```python
from build123d import *

# Parameters (mm, degrees)
BOSS_EXTRUDE1_DEPTH = 10.16
SKETCH5_W           = 63.5
SKETCH5_H           = 20.32
CUT_EXTRUDE1_DEPTH  = 2126.25967614


with BuildPart() as part:
    # Sketch1 → Boss-Extrude1 (new body)
    with BuildSketch(Plane.XY):
        Polygon((-123.444, 2072.64), (-205.715298803, 2072.64), (-205.715298803, 2052.32), (-215.881789204, 2052.32), (-215.881789204, 1963.42), (-205.715298803, 1963.42), (-205.715298803, 1874.52), (-215.881789204, 1874.52), (-215.881789204, 1785.62), (-205.715298803, 1785.62), (-205.715298803, 1696.72), (-215.875298803, 1696.72), (-215.875298803, 1607.82), (-205.715298803, 1607.82), (-205.715298803, 1518.92), (-215.881789204, 1518.92), (-215.881789204, 1488.440000035), (-469.881789204, 1488.440000035), (-469.881789204, 0), (-375.428294602, 0), (-375.428294602, 20.32), (-280.9748, 20.32), (-280.9748, 0), (280.9748, 0), (280.9748, 20.32), (375.428294602, 20.32), (375.428294602, 0), (469.881789204, 0), (469.881789204, 1488.440000035), (215.881789204, 1488.440000035), (215.881789204, 1518.92), (205.715298803, 1518.92), (205.715298803, 1607.82), (215.875298803, 1607.82), (215.875298803, 1696.72), (205.715298803, 1696.72), (205.715298803, 1785.62), (215.881789204, 1785.62), (215.881789204, 1874.52), (205.715298803, 1874.52), (205.715298803, 1963.42), (215.881789204, 1963.42), (215.881789204, 2052.32), (205.715298803, 2052.32), (205.715298803, 2072.64), (123.444, 2072.64), (123.444, 2052.32), (41.135649402, 2052.32), (41.135649402, 2072.64), (-41.135649402, 2072.64), (-41.135649402, 2052.32), (-123.444, 2052.32), align=None)
        Polygon((215.881789204, 1463.040000035), (222.040744894, 1374.366931824), (211.92306481, 1373.664189215), (205.715298803, 1463.040000035), align=None, mode=Mode.SUBTRACT)
        Polygon((-205.715298803, 1463.040000035), (-211.92306481, 1373.664189215), (-222.040744894, 1374.366931824), (-215.881789204, 1463.040000035), align=None, mode=Mode.SUBTRACT)
        Polygon((240.15668194, 1113.544188093), (246.676567651, 1019.674658983), (236.558887567, 1018.971916374), (230.039001856, 1112.841445484), align=None, mode=Mode.SUBTRACT)
        Polygon((-308.266124544, 132.94397688), (-301.755453134, 226.680843836), (-291.63777305, 225.978101227), (-298.14844446, 132.241234271), align=None, mode=Mode.SUBTRACT)
        Polygon((-289.435698895, 404.053512688), (-279.318018811, 403.350770078), (-285.830533081, 309.587370692), (-295.948213166, 310.290113301), align=None, mode=Mode.SUBTRACT)
        Polygon((-283.630301787, 487.636249721), (-277.115944656, 581.426181539), (-266.998264572, 580.72343893), (-273.512621703, 486.933507112), align=None, mode=Mode.SUBTRACT)
        Polygon((-264.796190418, 758.798850391), (-254.678510334, 758.096107781), (-261.194710324, 664.279643533), (-271.312390408, 664.982386142), align=None, mode=Mode.SUBTRACT)
        Polygon((-252.476436179, 936.171519242), (-242.358756095, 935.468776633), (-248.876798945, 841.625779953), (-258.99447903, 842.328522563), align=None, mode=Mode.SUBTRACT)
        Polygon((301.755453134, 226.680843836), (308.266124544, 132.94397688), (298.14844446, 132.241234271), (291.63777305, 225.978101227), align=None, mode=Mode.SUBTRACT)
        Polygon((279.318018811, 403.350770078), (289.435698895, 404.053512688), (295.948213166, 310.290113301), (285.830533081, 309.587370692), align=None, mode=Mode.SUBTRACT)
        Polygon((277.115944656, 581.426181539), (283.630301787, 487.636249721), (273.512621703, 486.933507112), (266.998264572, 580.72343893), align=None, mode=Mode.SUBTRACT)
        Polygon((254.678510334, 758.096107781), (264.796190418, 758.798850391), (271.312390408, 664.982386142), (261.194710324, 664.279643533), align=None, mode=Mode.SUBTRACT)
        Polygon((242.358756095, 935.468776633), (252.476436179, 936.171519242), (258.99447903, 842.328522563), (248.876798945, 841.625779953), align=None, mode=Mode.SUBTRACT)
        Polygon((-240.15668194, 1113.544188093), (-230.039001856, 1112.841445484), (-236.558887567, 1018.971916374), (-246.676567651, 1019.674658983), align=None, mode=Mode.SUBTRACT)
        Polygon((-227.836927701, 1290.916856945), (-217.719247617, 1290.214114336), (-224.240976188, 1196.318052795), (-234.358656272, 1197.020795404), align=None, mode=Mode.SUBTRACT)
        Polygon((217.719247617, 1290.214114336), (227.836927701, 1290.916856945), (234.358656272, 1197.020795404), (224.240976188, 1196.318052795), align=None, mode=Mode.SUBTRACT)
    extrude(amount=BOSS_EXTRUDE1_DEPTH)

    # Sketch5 → Cut-Extrude1 (cut, through all)
    with BuildSketch(Plane.XY.offset(10.16)):
        with Locations((-501.631789204, 10.16)):
            Rectangle(SKETCH5_W, SKETCH5_H)
        with Locations((501.631789204, 10.16)):
            Rectangle(SKETCH5_W, SKETCH5_H)
    extrude(amount=-CUT_EXTRUDE1_DEPTH, mode=Mode.SUBTRACT)


solid = part.part
```
CAD build for the part. Positions are in the model's coordinates, mm. Give positions to 0.01 mm unless a question says otherwise; leave off trailing zeros. Order: outer loops, then holes, each group sorted by start corner. A loop starts at its lowest first (then second) coordinate and runs counter-clockwise, first axis right, second up.
(1) Saw through at A-A, the plane y = 724. Give the cut face in (x, z).
(2) Drill centre lines: L1, parallel to X at y = 1286, z = 4.75; L2, parallel to X at y = 347.5, z = 4.75; L3, parallel to Y at x = 277, z = 1.5. Where is each one in solid material? Low to high.
(3) Flat gauge pins, fed straight in: pin 1 (3 mm diameter, centred on y = 1743, z = 5, fed in from +X); pin 2 (3 mm diameter, centred on y = 2006, z = 5, fed in from -X); pin 3 (3 mm diameter, centred on x = 295.5, z = 8.5, fed in from -Y). Where does each tip first touch, or does it go through?
(4) Saw through at B-B, the plane z = 5. State how many separate pieces and enclosed holes the cut face has, then the cut area to 3 significant figures.
(5) Saw through at D-D, the plane y = 1580. Give the cut face in (x, z).
(6) Saw through at C-C, the plane x = 404. Give the cut face in (y, z).
Results found:
1. outline: (-469.88, 0) - (-267.21, 0) - (-267.21, 10.16) - (-469.88, 10.16) - close; (-257.05, 0) - (257.05, 0) - (257.05, 10.16) - (-257.05, 10.16) - close; (267.21, 0) - (469.88, 0) - (469.88, 10.16) - (267.21, 10.16) - close
2. L1: x = -469.88 to -228.18, -218.01 to 218.01, 228.18 to 469.88
2. L2: x = -469.88 to -293.36, -283.2 to 283.2, 293.36 to 469.88
2. L3: y = 0 to 487.18, 581.42 to 1488.44
3. pin 1: stops at x = 205.72
3. pin 2: stops at x = -215.88
3. pin 3: stops at y = 20.32
4. separate pieces: 1
4. enclosed holes: 16
4. area: 1,620,000 mm2
5. outline: (-205.72, 0) - (205.72, 0) - (205.72, 10.16) - (-205.72, 10.16) - close
6. outline: (0, 0) - (1488.44, 0) - (1488.44, 10.16) - (0, 10.16) - close
